Source: CAD feature listing. Evaluate the final solid. Frame: model axes, mm. A direction names the side the tool comes from. Give positions to 0.01 mm unless a question says otherwise; leave off trailing zeros. Order: outer loops, then holes, each group sorted by start corner. A loop starts at its lowest first (then second) coordinate and runs counter-clockwise, first axis right, second up. Notation, with made-up numbers: (-31.5, 36) -> (23.5, 36) arc R20 ccw to (23.5, 54) -> close; hole circle Ø10 at (27.5, -34). An arc over 180 degrees is marked (long way). Answer in a Markdown table with one row per item.
```python
from build123d import *

# Parameters (mm, degrees)
F1_DEPTH = 84.7620591521
F2_R     = 7.5874829839
F3_DEPTH = 406.0934484005


# Not quite as in the source:
# - the program builds the solid bodies; features that only make, move or delete a surface that nothing else refers to are left out


with BuildPart() as f1:
    # F0 (on Top) → F1 (new body)
    with BuildSketch(Plane.XY):
        Polygon((29.4313300401, 27.8682895005), (-32.9063385725, 27.8682895005), (-30.3279589862, -28.8718193769), (29.4313300401, -28.8718193769), align=None)
    extrude(amount=-F1_DEPTH)

    # F2 (on Top) → F3 (join)
    with BuildSketch(Plane.XY):
        Circle(F2_R)
    extrude(amount=F3_DEPTH)


solid = f1.part
```
(1) Access query for faces 1 (the cylindrical face through (4.079, 6.398, 200.204)), 2 (the flat face through (-31.635, -0.105, -41.788)). Directions: +Z, -Z, +X, -X, +Y, -Y. A direction counts if a zero-diameter tool reaches every point of the face in a straight line with its end or side. Return the directions, or none.
A:
| item | result |
|---|---|
| face 1 | +Z |
| face 2 | +Z, -Z, -X, -Y |
(2) Section query D-D (x = -25). Return the cut outline in (y, z).
A:
| item | result |
|---|---|
| outline | (-28.87, -84.76) -> (27.87, -84.76) -> (27.87, 0) -> (-28.87, 0) -> close |
(3) Section query B-B (z = 168.5). Return the cut outline in (x, y).
A:
| item | result |
|---|---|
| outline | circle Ø15.17 at (0, 0) |
(4) Section query A-A (x = 0). Return the cut outline in (y, z).
A:
| item | result |
|---|---|
| outline | (-28.87, -84.76) -> (27.87, -84.76) -> (27.87, 0) -> (7.59, 0) -> (7.59, 406.09) -> (-7.59, 406.09) -> (-7.59, 0) -> (-28.87, 0) -> close |
(5) Ray query, probe 1 along Z at (x, y) = (-11.5, -4.5); probe 2 along X at (y, z) = (5, 268); probe 3 along X at (y, z) = (-5.5, 119). Return the intervals inside material, ascending.
A:
| item | result |
|---|---|
| probe 1 | z = -84.76 to 0 |
| probe 2 | x = -5.71 to 5.71 |
| probe 3 | x = -5.23 to 5.23 |
(6) Section query C-C (y = 0). Return the cut outline in (x, z), plus the area to 3 significant figures.
A:
| item | result |
|---|---|
| outline | (-31.64, -84.76) -> (29.43, -84.76) -> (29.43, 0) -> (7.59, 0) -> (7.59, 406.09) -> (-7.59, 406.09) -> (-7.59, 0) -> (-31.64, 0) -> close |
| area | 11,300 mm^2 |
(7) First-contact query: pin 1 Ø17 at (x, y) = (8.5, 5) entering from +Z; pin 2 Ø1.5 at (x, z) = (4.5, 66.5) entering from -Y; pin 3 Ø3 at (x, z) = (-1, 147) entering from -Y; pin 4 Ø3 at (y, z) = (4, 85) entering from -X. Flat tips, straight axial feed; report the tip coordinate or a pass-through.
A:
| item | result |
|---|---|
| pin 1 | stops at z = 406.09 |
| pin 2 | stops at y = -6.6 |
| pin 3 | stops at y = -7.59 |
| pin 4 | stops at x = -7.16 |
